The drawing under review shows one solid part. Ordinate dimensions are in mm from its lowest x, y, z. A direction names the side the tool comes from. Round coordinates to 2 decimals unless told otherwise and drop trailing zeros. Loops run counter-clockwise (first coordinate to the right, second up) from the corner with the lowest first, then second, coordinate; pieces in that order, holes last. Notation, with made-up numbers: M -20.5,10.5 L -3.5,10.5 A13 cw -3.5,15.5 Z; hole C 0,-8 d3. An arc over 180 degrees is marked long. Use a Markdown table: item, result.
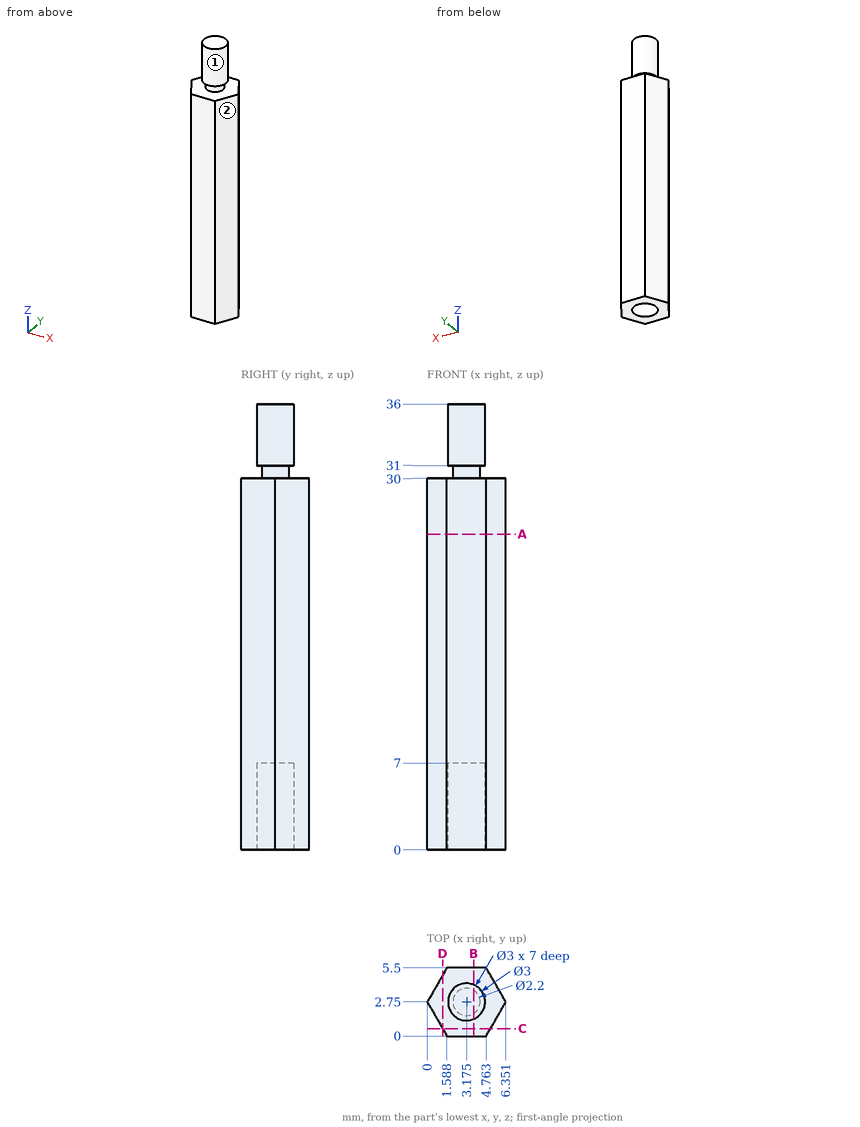
1. Take a section at D-D on x = 1.25. Give the boundary of the cut face in (y, z) (1 decimal).
Check values:
| item | result |
|---|---|
| outline | M 0.6,0 L 4.9,0 L 4.9,30 L 0.6,30 Z |
2. Take a section at C-C on y = 0.6. Give the boundary of the cut face in (x, z).
Check values:
| item | result |
|---|---|
| outline | M 1.24,0 L 5.11,0 L 5.11,30 L 1.24,30 Z |
3. Take a section at A-A on z = 25.5. Give the boundary of the cut face in (x, y), and give its area (3 significant figures).
Check values:
| item | result |
|---|---|
| outline | M 0,2.75 L 1.59,0 L 4.76,0 L 6.35,2.75 L 4.76,5.5 L 1.59,5.5 Z |
| area | 26.2 mm² |
4. Insertion check: pin 1 (1 mm diameter, centred on x = 2, y = 4.5, fed in from +Z). The pin has a flat end and moves straight along its axis. Give the tip position at first contact, or say it passes through.
Check values:
| item | result |
|---|---|
| pin 1 | stops at z = 30 |
5. Take a section at B-B on x = 3.75. Give the boundary of the cut face in (y, z) (1 decimal).
Check values:
| item | result |
|---|---|
| outline | M 0,0 L 1.4,0 L 1.4,7 L 4.1,7 L 4.1,0 L 5.5,0 L 5.5,30 L 3.7,30 L 3.7,31 L 4.1,31 L 4.1,36 L 1.4,36 L 1.4,31 L 1.8,31 L 1.8,30 L 0,30 Z |
6. Wall thickness on line 1 along Z through (x, y) = (4.75, 2.05); line 2 along Z through (x, y) = (4, 1.6); line 3 along Z through (x, y) = (3.5, 3.5): over which ranges is each line inside the solid? List them lowest first. Write a range as from..to.
Check values:
| item | result |
|---|---|
| line 1 | z = 0..30 |
| line 2 | z = 7..30, 31..36 |
| line 3 | z = 7..36 |
7. Machinability: for the marked faces 1 and 2, which of the approach directions +Z, -Z, +X, -X, +Y, -Y give a long, thin tool a straight path to every point of the face, cutting with its end or side? Answer none if there is none.
Check values:
| item | result |
|---|---|
| face 1 | +Z |
| face 2 | +Z, -Z, +X, -Y |
